CAD build for the part. Positions are in the model's coordinates, mm. A direction names the side the tool comes from. Round coordinates to 2 decimals unless told otherwise and drop trailing zeros. Order: outer loops, then holes, each group sorted by start corner. A loop starts at its lowest first (then second) coordinate and runs counter-clockwise, first axis right, second up. Notation, with made-up numbers: M -8,-29.5 L 16,-29.5 A12 ccw 16,-14.5 Z; hole C -4,-32 d6. An arc over 180 degrees is marked long. Answer as a JSON object with one key per item and string values. Group by question number.
Autodesk Inventor part; units mm, degrees
ref_plane "Płaszczyzna konstrukcyjna1" through (10, 8.2, 0) normal (1, 0, 0) x (0, 0, -1)
ref_plane "YZ Plane" through (0, 0, 0) normal (1, 0, 0) x (0, 1, 0)
ref_plane "XZ Plane" through (0, 0, 0) normal (0, 1, 0) x (-1, 0, 0)
sketch "Szkic1" plane through (0, 0, 0) normal (0, 0, 1) x (1, 0, 0)
  circle A0 centre (0, 0) radius 2.1
  line L0 (-10, 10) -> (10, 10)
  line L1 (10, 10) -> (10, -10)
  line L2 (10, -10) -> (-10, -10)
  line L3 (-10, -10) -> (-10, 10)
  line L4 (-10, -10) -> (10, 10) construction
  line L5 (10, -10) -> (-10, 10) construction
  line L6 (-10, 8.2) -> (10, 8.2)
  line L7 (-10, -8.2) -> (10, -8.2)
  line L8 (-8.2, 10) -> (-8.2, -10)
  line L9 (10, 10) -> (30, 10)
  line L10 (30, 10) -> (30, -10)
  line L11 (30, -10) -> (10, -10)
  line L12 (10, -10) -> (10, 10)
  line L13 (-4.1857, -4.1857) -> (4.1857, -4.1857)
  line L14 (4.1857, -4.1857) -> (4.1857, 4.1857)
  line L15 (4.1857, 4.1857) -> (-4.1857, 4.1857)
  line L16 (-4.1857, 4.1857) -> (-4.1857, -4.1857)
  line L17 (-8.2, 7.1393) -> (-4.1857, 3.125)
  line L18 (-7.1393, 8.2) -> (-3.125, 4.1857)
  line L19 (-4.925, 10) -> (-3.125, 8.2)
  line L20 (4.925, 10) -> (3.125, 8.2)
  line L21 (-3.125, -8.2) -> (-4.925, -10)
  line L22 (3.125, -8.2) -> (4.925, -10)
  line L23 (-8.2, -7.1393) -> (-4.1857, -3.125)
  line L24 (-7.1393, -8.2) -> (-3.125, -4.1857)
  line L25 (3.125, -4.1857) -> (7.1393, -8.2)
  line L26 (4.1857, -3.125) -> (7.3007, -6.24)
  line L27 (4.1857, 3.125) -> (7.3007, 6.24)
  line L28 (3.125, 4.1857) -> (7.1393, 8.2)
  line L29 (-5.4993, 8.2) -> (-5.4993, 6.56)
  line L30 (5.4993, 8.2) -> (5.4993, 6.56)
  line L31 (-8.2, 5.4993) -> (-6.56, 5.4993)
  line L32 (-8.2, -5.4993) -> (-6.56, -5.4993)
  line L33 (-5.4993, -6.56) -> (-5.4993, -8.2)
  line L34 (5.4993, -6.56) -> (5.4993, -8.2)
  line L35 (-8.2, 3.125) -> (-10, 4.925)
  line L36 (-8.2, -3.125) -> (-10, -4.925)
  line L37 (7.3007, 6.24) -> (7.3007, 8.2)
  line L38 (7.3007, -6.24) -> (7.3007, -8.2)
  point P0 (0, -8.2)
  point P1 (-8.2, -8.2)
  point P2 (-8.2, 8.2)
  dimension "d0" = 4.2
  dimension "d1" = 20
  dimension "d2" = 1.8
  dimension "d4" = 20
  dimension "d5" = 20
  dimension "d6" = 1.8
  dimension "d7" = 1.8
  dimension "d8" = 1.5
  dimension "d9" = 0.75
  dimension "d10" = 135
  dimension "d11" = 6.25
  dimension "d12" = 3.125
  dimension "d13" = 1.5
  dimension "d14" = 1.5
  dimension "d15" = 1.5
  dimension "d16" = 0.75
  dimension "d17" = 0.75
  dimension "d18" = 0.75
  dimension "d19" = 1.64
  dimension "d20" = 1.64
  dimension "d21" = 1.64
  dimension "d22" = 1.64
  dimension "d23" = 1.64
  dimension "d24" = 1.64
  dimension "d25" = 45
  dimension "d30" = 1.96
  dimension "d31" = 1.96
extrude "Wyciągnięcie proste1" add sketch "Szkic1" along normal blind 120 contours L0 L8 L6 L3 | L0 L19 L6 L8 | L6 L8 L35 L3 | L6 L18 L15 L16 L17 L8 | L0 L1 L6 L20 | L6 L29 L18 | L17 L31 L8 | L36 L8 L7 L3 | L7 L8 L2 L3 | L6 L28 L30 | L15 L14 L13 L16 | L8 L23 L16 L13 L24 L7 | L7 L21 L2 L8 | L32 L23 L8 | L1 L2 L22 L7 | L37 L27 L14 L15 L28 L6 | L24 L33 L7 | L7 L25 L13 L14 L26 L38 | L7 L34 L25
ref_plane "Płaszczyzna konstrukcyjna1" through (10, 8.2, 0) normal (1, 0, 0) x (0, 0, -1)
mirror "Odbij1" about plane through (10, 8.2, 0) normal (1, 0, 0) of "Wyciągnięcie proste1"
fillet "Zaokrąglenie1" radius 0.5 4 edges at (-10, 10, 60) (-10, -10, 60) (30, 10, 60) (30, -10, 60)
properties part number "2040vslot_short"
Item 1: Cut at C-C, the plane z = 23. Give the number of separate pieces and of enclosed holes in the cut face, and give its area (3 significant figures).
Item 2: Cut at B-B, the plane y = 0. Give the cut face in (x, z), and give its area (3 significant figures).
Item 3: Cut at A-A, the plane x = 0. Give the cut face in (y, z), and give its area (3 significant figures).
Item 4: Flat gauge pins, fed straight in: pin 1 Ø1.2 at (x, z) = (4, 68) entering from -Y (3 decimals); pin 2 Ø5 at (x, z) = (19.5, 69) entering from -Y; pin 3 Ø0.7 at (x, z) = (15.5, 36) entering from +Y (3 decimals). Where does each tip first touch, or does it go through?
Item 5: 3-axis set-ups, long thin cutter, end or side, ignore diameter. For faces 4 (the face through (0, -4.186, 59)), 5 (the face through (4.3, 5.36, 59.16)), 6 (the face through (0, 4.186, 59)): which of +Z, -Z, +X, -X, +Y, -Y reach the whole face in a straight line?
Item 6: Drill centre lines: line 1 (Y direction, x = 0, z = 45); line 2 (Y direction, x = -5, z = 22); line 3 (X direction, y = -8.5, z = 17) (3 decimals). Where is each one in solid material? Low to high. Write a range as [from, to].
Item 7: Two-plate mould, pull along X, no slides. Class faces 1 (the face through (7.301, -7, 59)), 2 (the face through (-10, 7, 59)), 3 (the face through (30, 7, 59)): +X half, -X half, draft (parallel to the pull), parting line (faces both ways), or undercut.
Response values:
{
 "1": {"separate pieces": "1", "enclosed holes": "3", "area": "307 mm^2"},
 "2": {"outline": "M -4.19,0 L -2.1,0 L -2.1,120 L -4.19,120 Z; M 2.1,0 L 4.19,0 L 4.19,120 L 2.1,120 Z; M 15.81,0 L 17.9,0 L 17.9,120 L 15.81,120 Z; M 22.1,0 L 24.19,0 L 24.19,120 L 22.1,120 Z", "area": "1,000 mm^2"},
 "3": {"outline": "M -4.19,0 L -2.1,0 L -2.1,120 L -4.19,120 Z; M 2.1,0 L 4.19,0 L 4.19,120 L 2.1,120 Z", "area": "501 mm^2"},
 "4": {"pin 1": "y = -9.675", "pin 2": "y = -4.19", "pin 3": "y = 9.925"},
 "5": {"face 4": "+Z, -Z, -Y", "face 5": "+Z, -Z", "face 6": "+Z, -Z, +Y"},
 "6": {"line 1": "[-4.19, -2.1], [2.1, 4.19]", "line 2": "[-10, -8.2], [-6.06, -3.94], [3.94, 6.06], [8.2, 10]", "line 3": "[-10, -3.425], [3.425, 16.575], [23.425, 30]"},
 "7": {"face 1": "undercut", "face 2": "-X half", "face 3": "+X half"}
}
